```python
from build123d import *

# Parameters (mm, degrees)
SKETCH_2_R      = 40
SKETCH_2_R_2    = 2.25
SKETCH_2_R_3    = 23
EXTRUDE_1_DEPTH = 3
SKETCH_3_R      = 40
SKETCH_3_R_2    = 4
SKETCH_3_R_3    = 23
EXTRUDE_2_DEPTH = 4
CHAMFER_1_SIZE  = 3
CHAMFER_2_SIZE  = 1


with BuildPart() as part:
    # ｽｹｯﾁ2 → ﾎﾞｽ - 押し出し1 (new body)
    with BuildSketch(Plane.XY):
        Circle(SKETCH_2_R)
        with Locations((0, 32)):
            Circle(SKETCH_2_R_2, mode=Mode.SUBTRACT)
        Circle(SKETCH_2_R_3, mode=Mode.SUBTRACT)
        with Locations((-27.712812921, 16)):
            Circle(SKETCH_2_R_2, mode=Mode.SUBTRACT)
        with Locations((-27.712812921, -16)):
            Circle(SKETCH_2_R_2, mode=Mode.SUBTRACT)
        with Locations((0, -32)):
            Circle(SKETCH_2_R_2, mode=Mode.SUBTRACT)
        with Locations((27.712812921, -16)):
            Circle(SKETCH_2_R_2, mode=Mode.SUBTRACT)
        with Locations((27.712812921, 16)):
            Circle(SKETCH_2_R_2, mode=Mode.SUBTRACT)
    extrude(amount=EXTRUDE_1_DEPTH)

    # ｽｹｯﾁ3 → ﾎﾞｽ - 押し出し2 (add)
    with BuildSketch(Plane.XY.offset(3)):
        Circle(SKETCH_3_R)
        with Locations((0, 32)):
            Circle(SKETCH_3_R_2, mode=Mode.SUBTRACT)
        with Locations((-27.712812921, 16)):
            Circle(SKETCH_3_R_2, mode=Mode.SUBTRACT)
        with Locations((-27.712812921, -16)):
            Circle(SKETCH_3_R_2, mode=Mode.SUBTRACT)
        with Locations((0, -32)):
            Circle(SKETCH_3_R_2, mode=Mode.SUBTRACT)
        with Locations((27.712812921, -16)):
            Circle(SKETCH_3_R_2, mode=Mode.SUBTRACT)
        with Locations((27.712812921, 16)):
            Circle(SKETCH_3_R_2, mode=Mode.SUBTRACT)
        Circle(SKETCH_3_R_3, mode=Mode.SUBTRACT)
    extrude(amount=EXTRUDE_2_DEPTH)

    # 面取り1
    chamfer_1_edges = [part.edges().sort_by_distance(p)[0] for p in [
        (-40, 0, 7),
    ]]
    chamfer(chamfer_1_edges, length=CHAMFER_1_SIZE)

    # 面取り2
    chamfer_2_edges = [part.edges().sort_by_distance(p)[0] for p in [
        (-23, 0, 7),
    ]]
    chamfer(chamfer_2_edges, length=CHAMFER_2_SIZE)


solid = part.part
```
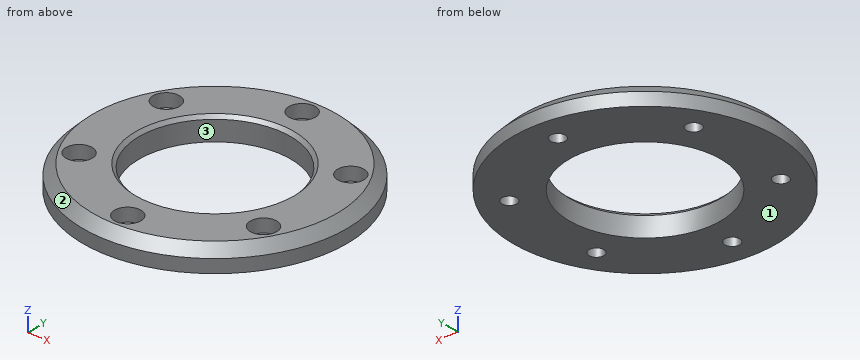
Source: CAD feature listing. Evaluate the final solid. Frame: model axes, mm. Face numbers are marked on the shaded views. Give positions to 0.01 mm unless a question says otherwise; leave off trailing zeros. Write each loop counter-clockwise with the first axis right and the second up, starting at its lowest first coordinate (ties: lowest second). Pieces come first, ordered by that corner, then holes. Notation, with made-up numbers: (89, -25) - (106, -25) arc R18 ccw to (106, -19) - close; hole circle Ø1 at (-8.5, 30). An arc over 180 degrees is marked (long way). One line per item, written item: value. Start each with the question number.
Q1. Draft query along Y for the marked faces 1, 2 and 3. Return one class per face: +Y half, -Y half, draft (parallel to the pull), parting line (faces both ways), or undercut.
Q2. First-contact query: pin 1 Ø5 at (x, y) = (27.71, 16) entering from -Z; pin 2 Ø2.5 at (x, y) = (28, -17.5) entering from +Z; pin 3 Ø2 at (y, z) = (-22, 3.5) entering from +X; pin 4 Ø3 at (y, z) = (-25, 1) entering from +X. Flat tips, straight axial feed; report the tip coordinate or a pass-through.
Q3. Material intervals for probe 1 along Y at (x, z) = (0, 2.35); probe 2 along Y at (x, z) = (-1, 4.25); probe 3 along Y at (x, z) = (28, 0.75), sorted ascending. Write a range as from..to.
Q4. Section query B-B, the plane x = 0. Return the cut outline in (y, z).
Q5. Section query A-A, the plane y = 0. Return the cut outline in (x, z), then the cut area to 3 significant figures.
Q6. Section query C-C, the plane y = 16. Count the separate pieces of the cut face and the enclosed holes in it, then the cut area to 3 significant figures.
Answer:
1. face 1: draft
1. face 2: parting line
1. face 3: undercut
2. pin 1: stops at z = 0
2. pin 2: stops at z = 3
2. pin 3: stops at x = 34.04
2. pin 4: stops at x = 32.37
3. probe 1: y = -40..-34.25, -29.75..-23, 23..29.75, 34.25..40
3. probe 2: y = -39.74..-35.87, -28.13..-22.98, 22.98..28.13, 35.87..39.74
3. probe 3: y = -28.57..-18.23, -13.77..13.77, 18.23..28.57
4. outline: (-40, 0) - (-34.25, 0) - (-34.25, 3) - (-36, 3) - (-36, 7) - (-37, 7) - (-40, 4) - close; (-29.75, 0) - (-23, 0) - (-23, 6) - (-24, 7) - (-28, 7) - (-28, 3) - (-29.75, 3) - close; (23, 0) - (29.75, 0) - (29.75, 3) - (28, 3) - (28, 7) - (24, 7) - (23, 6) - close; (34.25, 0) - (40, 0) - (40, 4) - (37, 7) - (36, 7) - (36, 3) - (34.25, 3) - close
5. outline: (-40, 0) - (-23, 0) - (-23, 6) - (-24, 7) - (-37, 7) - (-40, 4) - close; (23, 0) - (40, 0) - (40, 4) - (37, 7) - (24, 7) - (23, 6) - close
5. area: 228 mm2
6. separate pieces: 4
6. enclosed holes: 0
6. area: 180 mm2
